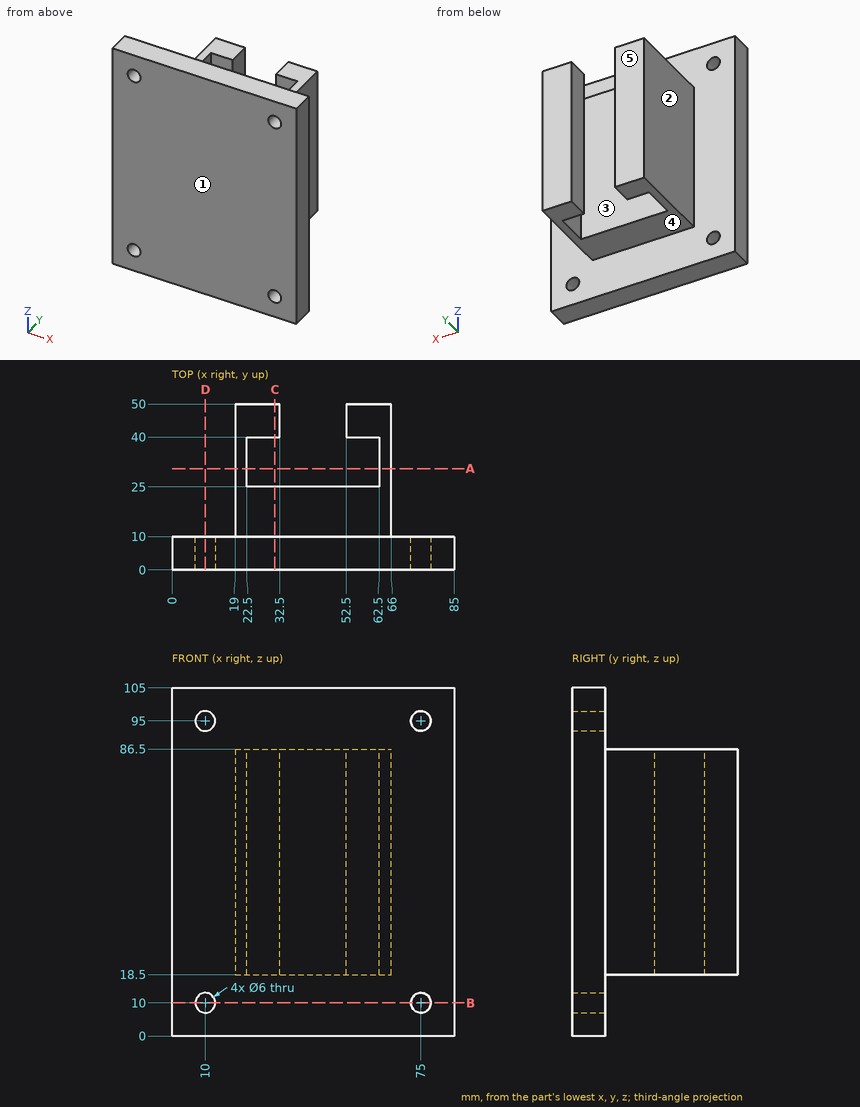
Study the drawing (mm; zero at the part's minimum x, y, z) and answer. A direction names the side the tool comes from. Give positions to 0.01 mm unless a question says otherwise; leave off trailing zeros. Write each loop counter-clockwise with the first axis right and the second up, starting at its lowest first coordinate (ties: lowest second). Pieces come first, ordered by that corner, then holes.
(1) The part is cut by section B-B on z = 10. Write down the section's boundary in (x, y).
Final values:
outline: (0, 0) - (7, 0) - (7, 10) - (0, 10) - close; (13, 0) - (72, 0) - (72, 10) - (13, 10) - close; (78, 0) - (85, 0) - (85, 10) - (78, 10) - close
(2) Which of the six approach directions +Z, -Z, +X, -X, +Y, -Y give full straight-line access (tool end or side, diameter ignored) to the marked faces 4 and 5?
Final values:
face 4: -Z, +X, -X, +Y
face 5: +Z, -Z, +X, -X, +Y
(3) Flat-ended cylindrical pins translate along their axes: pin 1 Ø12 at (y, z) = (31.5, 44) entering from -X; pin 2 Ø4 at (x, y) = (17.5, 38) entering from -Z; pin 3 Ø4.5 at (y, z) = (33, 62.5) entering from +X. Find the tip coordinate at first contact, or state that the pin passes through.
Final values:
pin 1: stops at x = 19
pin 2: stops at z = 18.5
pin 3: stops at x = 66
(4) The part is cut by section A-A on y = 30.5. Write down the section's boundary in (x, z).
Final values:
outline: (19, 18.5) - (22.5, 18.5) - (22.5, 86.5) - (19, 86.5) - close; (62.5, 18.5) - (66, 18.5) - (66, 86.5) - (62.5, 86.5) - close
(5) The mould has two halves that part along Y. Classify the marked faces 1, 2 and 3: pulls with the +Y half, pulls with the -Y half, needs draft (parallel to the pull), parting line crosses it, or undercut.
Final values:
face 1: pulls with the -Y half
face 2: needs draft
face 3: undercut
(6) The part is cut by section D-D on x = 10. Write down the section's boundary in (y, z).
Final values:
outline: (0, 0) - (10, 0) - (10, 7) - (0, 7) - close; (0, 13) - (10, 13) - (10, 92) - (0, 92) - close; (0, 98) - (10, 98) - (10, 105) - (0, 105) - close
(7) Straight lines are drawn through the part: line 1 (Z direction, x = 10, y = 4.75); line 2 (X direction, y = 47, z = 69); line 3 (X direction, y = 32.5, z = 65.5). For each, find the intervals that lie inside material, in ascending order.
Final values:
line 1: z = 0 to 7, 13 to 92, 98 to 105
line 2: x = 19 to 32.5, 52.5 to 66
line 3: x = 19 to 22.5, 62.5 to 66
(8) The part is cut by section C-C on x = 31. Write down the section's boundary in (y, z), plus the area to 3 significant figures.
Final values:
outline: (0, 0) - (10, 0) - (10, 18.5) - (25, 18.5) - (25, 86.5) - (10, 86.5) - (10, 105) - (0, 105) - close; (40, 18.5) - (50, 18.5) - (50, 86.5) - (40, 86.5) - close
area: 2,750 mm2
